Check sheet for the modelled part. Datum: model origin and axes. Units: mm. Face numbers are marked on the shaded views. Round coordinates to 2 decimals unless told otherwise and drop trailing zeros. Write each loop counter-clockwise with the first axis right and the second up, starting at its lowest first coordinate (ties: lowest second). Pieces come first, ordered by that corner, then holes. Notation, with made-up numbers: M -4,-6.75 L 51,-6.75 A11 cw 51,7.25 Z; hole C 87.25,20 d10. An arc over 180 degrees is marked long. Put each result on its own line as item: value.
```python
from build123d import *

# Parameters (mm, degrees)
F1_DEPTH = 12.7
F2_R     = 14.718879
F3_DEPTH = 22.605523
F4_R     = 5.08


with BuildPart() as f1:
    # F0 (on Front) → F1 (new body, symmetric)
    with BuildSketch(Plane.XZ):
        Polygon((-28.836578, 0), (0, 0), (26.969403, 0), (0, 37.134841), align=None)
    extrude(amount=F1_DEPTH, both=True)

    # F2 (on Front) → F3 (cut, symmetric)
    with BuildSketch(Plane.XZ):
        Circle(F2_R)
    extrude(amount=F3_DEPTH, both=True, mode=Mode.SUBTRACT)

    # F4
    f4_edges = [f1.edges().sort_by_distance(p)[0] for p in [
        (0, 0, 37.134841),
    ]]
    fillet(f4_edges, radius=F4_R)


solid = f1.part
```
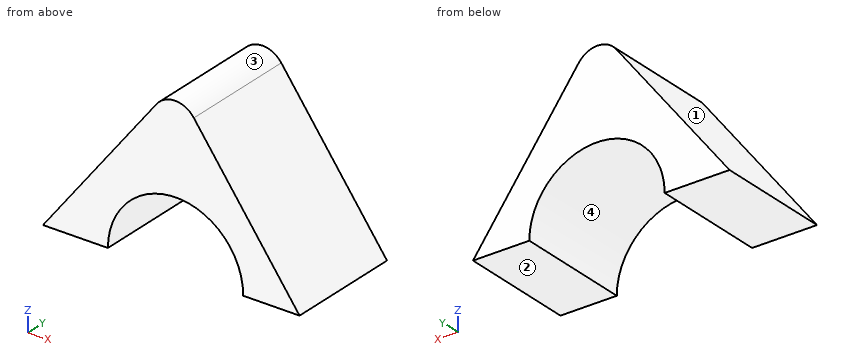
1. Cross-section at A-A (z = 5.5). Enter the section's corners in (x, y) (3 decimals), then the cut area to 3 significant figures.
Computed values:
outline: M -24.566,-12.7 L -13.653,-12.7 L -13.653,12.7 L -24.566,12.7 Z; M 13.653,-12.7 L 22.975,-12.7 L 22.975,12.7 L 13.653,12.7 Z
area: 514 mm2
2. Cross-section at D-D (z = 18). Enter the section's corners in (x, y).
Computed values:
outline: M -14.86,-12.7 L 13.9,-12.7 L 13.9,12.7 L -14.86,12.7 Z
3. Cross-section at B-B (y = 9.75). Enter the section's corners in (x, z).
Computed values:
outline: M -28.84,0 L -14.72,0 A14.72 cw 14.72,0 L 26.97,0 L 3.97,31.66 A5.08 ccw -4.15,31.79 Z
4. Cross-section at C-C (x = 0). Enter the section's corners in (y, z), then the cut area to 3 significant figures.
Computed values:
outline: M -12.7,14.72 L 12.7,14.72 L 12.7,33.76 L -12.7,33.76 Z
area: 484 mm2
5. Release check for a two-part mould opening along X. For the marked faces 1, 2, 3 and 4 record: +X half, -X half, draft (parallel to the pull), parting line (faces both ways), or undercut.
Computed values:
face 1: -X half
face 2: draft
face 3: parting line
face 4: undercut
6. Scan lines: probe 1 along X at (y, z) = (11.75, 5.5) (3 decimals); probe 2 along Z at (x, y) = (0, 1.25); probe 3 along X at (y, z) = (-2.5, 3). Record each from-to range of solid material in increasing order.
Computed values:
probe 1: x = -24.566 to -13.653, 13.653 to 22.975
probe 2: z = 14.72 to 33.76
probe 3: x = -26.51 to -14.41, 14.41 to 24.79
7. Depth check by flat-ended pin: pin 1 Ø12 at (y, z) = (-1.5, 20.5) entering from -X; pin 2 Ø1.5 at (y, z) = (4, 20) entering from -X; pin 3 Ø3 at (y, z) = (3.5, 13.5) entering from -X. Enter the tip coordinate at first touch or a pass-through.
Computed values:
pin 1: stops at x = -17.58
pin 2: stops at x = -13.89
pin 3: stops at x = -19.52
